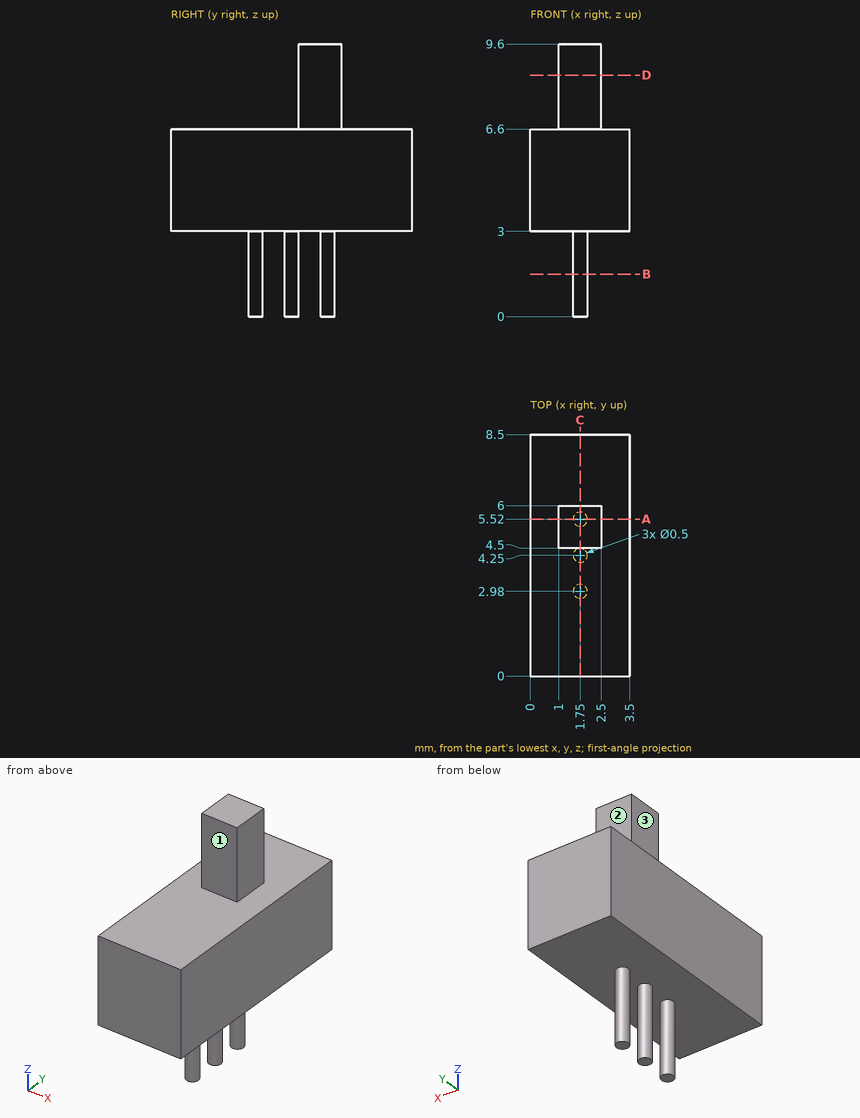
Verification items for this drawing (mm, ordinates from the low corner). A direction names the side the tool comes from. Coordinates: 2 decimals unless noted, no trailing zeros. Order: outer loops, then holes, each group sorted by start corner. A loop starts at its lowest first (then second) coordinate and runs counter-clockwise, first axis right, second up.
Q1. Tool access check on the marked faces 1, 2 and 3. Record the directions out of +Z, -Z, +X, -X, +Y, -Y that give a thin tool (end or side, any length) a straight path to the whole face; none if there is none.
Reply:
face 1: +Z, +X, -X, -Y
face 2: +Z, +X, -X, +Y
face 3: +Z, -X, +Y, -Y
Q2. Sectioned sample at B-B on z = 1.5. Record the cut outline in (x, y).
Reply:
outline: circle Ø0.5 at (1.75, 2.98); circle Ø0.5 at (1.75, 4.25); circle Ø0.5 at (1.75, 5.52)
Q3. Sectioned sample at C-C on x = 1.75. Record the cut outline in (y, z), and give its area (3 significant figures).
Reply:
outline: (0, 3) - (2.73, 3) - (2.73, 0) - (3.23, 0) - (3.23, 3) - (4, 3) - (4, 0) - (4.5, 0) - (4.5, 3) - (5.27, 3) - (5.27, 0) - (5.77, 0) - (5.77, 3) - (8.5, 3) - (8.5, 6.6) - (6, 6.6) - (6, 9.6) - (4.5, 9.6) - (4.5, 6.6) - (0, 6.6) - close
area: 39.6 mm2
Q4. Thickness scan on probe 1 along Y at (x, z) = (1.85, 0.5); probe 2 along Z at (x, y) = (1.05, 4.25); probe 3 along Z at (x, y) = (2.1, 5). Record the ranges inside material, lowest first.
Reply:
probe 1: y = 2.75 to 3.21, 4.02 to 4.48, 5.29 to 5.75
probe 2: z = 3 to 6.6
probe 3: z = 3 to 9.6
Q5. Depth check by flat-ended pin: pin 1 Ø1 at (x, y) = (2, 1.5) entering from -Z; pin 2 Ø1.6 at (y, z) = (5.5, 8) entering from +X; pin 3 Ø1.6 at (y, z) = (5, 7.5) entering from -X. Enter the tip coordinate at first touch or a pass-through.
Reply:
pin 1: stops at z = 3
pin 2: stops at x = 2.5
pin 3: stops at x = 1
Q6. Sectioned sample at A-A on y = 5.52. Record the cut outline in (x, z), and give its area (3 significant figures).
Reply:
outline: (0, 3) - (1.5, 3) - (1.5, 0) - (2, 0) - (2, 3) - (3.5, 3) - (3.5, 6.6) - (2.5, 6.6) - (2.5, 9.6) - (1, 9.6) - (1, 6.6) - (0, 6.6) - close
area: 18.6 mm2
Q7. Sectioned sample at D-D on z = 8.5. Record the cut outline in (x, y).
Reply:
outline: (1, 4.5) - (2.5, 4.5) - (2.5, 6) - (1, 6) - close
